Geometry check sheet. Reference: drawing and pictorial views, mm from the part's lowest x, y, z. Round coordinates to 2 decimals unless told otherwise and drop trailing zeros. Order: outer loops, then holes, each group sorted by start corner. A loop starts at its lowest first (then second) coordinate and runs counter-clockwise, first axis right, second up.
(1) Sectioned sample at B-B, the plane y = 5. Enter the section's corners in (x, z), and give its area (3 significant figures).
(2) Depth check by flat-ended pin: pin 1 (2 mm diameter, centred on y = 60.5, z = 32, fed in from -X); pin 2 (2 mm diameter, centred on x = 1.5, z = 25, fed in from -Y); pin 3 (0.8 mm diameter, centred on x = 88.5, z = 30.5, fed in from -Y); pin 4 (12 mm diameter, centred on x = 70, y = 60, fed in from -Z). Enter the tip coordinate at first touch or a pass-through.
(3) Thickness scan on probe 1 along X at (y, z) = (38.5, 28); probe 2 along Y at (x, z) = (59, 43.5); probe 3 along Z at (x, y) = (13.5, 6). Record the ranges inside material, lowest first.
(4) Mould release check, pull along Z, two halves, no side actions. Record for the marked faces 1, 2 and 3: released by +Z, released by -Z, zero draft, split by the parting line, or undercut.
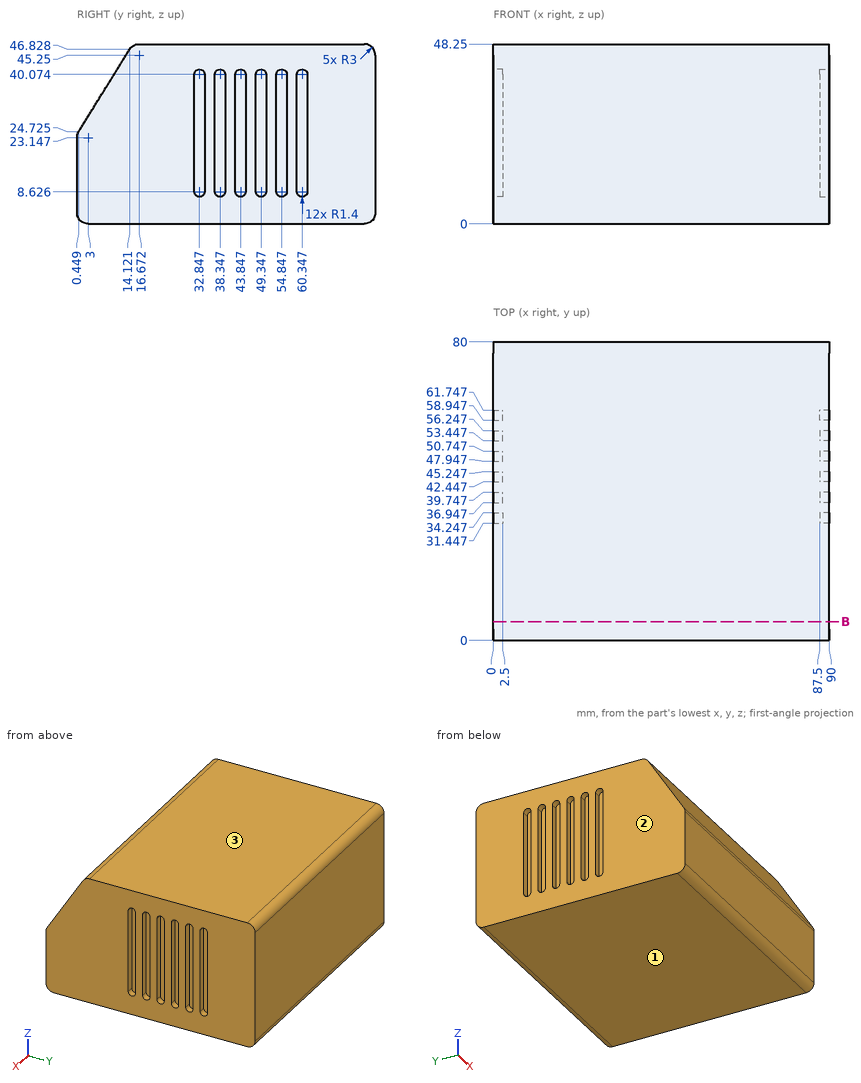
Derived:
1. outline: (0, 0) - (90, 0) - (90, 32.08) - (0, 32.08) - close
1. area: 2,890 mm2
2. pin 1: stops at x = 2.5
2. pin 2: stops at y = 0.12
2. pin 3: stops at y = 3.77
2. pin 4: stops at z = 0
3. probe 1: x = 2.5 to 87.5
3. probe 2: y = 12.06 to 80
3. probe 3: z = 0 to 33.7
4. face 1: released by -Z
4. face 2: zero draft
4. face 3: released by +Z
